Geometry: see drawing. Coordinates: mm, zero at the bounding-box minimum. A direction names the side the tool comes from. Coordinates: 2 decimals unless noted, no trailing zeros. Write each loop counter-clockwise with the first axis right and the second up, starting at its lowest first coordinate (ties: lowest second). Pieces come first, ordered by that corner, then holes. Notation, with made-up numbers: M 85.5,31.25 L 98.5,31.25 A17 cw 98.5,46.25 Z; hole C 89.25,33 d10. An arc over 180 degrees is marked long. Answer as CSV lines item,"result". Start each with the question number.
1. Section B-B on y = 70. Return the cut outline in (x, z), plus the area to 3 significant figures.
2. Contact query for flat-ended pins moving along their axis: pin 1 Ø2 at (x, z) = (172.5, 100) entering from +Y; pin 2 Ø10 at (x, z) = (100.5, 121.5) entering from +Y. Output: stop coordinate, or through.
3. Section D-D on z = 123.5. Return the cut outline in (x, y), plus the area to 3 significant figures.
4. Reachability of the marked faces 1 and 2 from +Z, -Z, +X, -X, +Y, -Y: full face, straight path, thin tool, end or side. Return the list, or none.
5. Mould query, pull axis Z, two halves, no side actions, for the marked faces 3, 4, 5 and 6. Classes: pulls with the +Z half, pulls with the -Z half, needs draft (parallel to the pull), parting line crosses it, or undercut.
6. Section C-C on z = 88.9. Return the cut outline in (x, y).
7. Line query: probe 1 along X at (y, z) = (24, 88); probe 2 along Z at (x, y) = (192, 61); probe 3 along Z at (x, y) = (215, 23). Output: solid intervals per line, ascending. Write a range as [from, to].
8. Section A-A on x = 88.9. Return the cut outline in (y, z), plus the area to 3 significant figures.
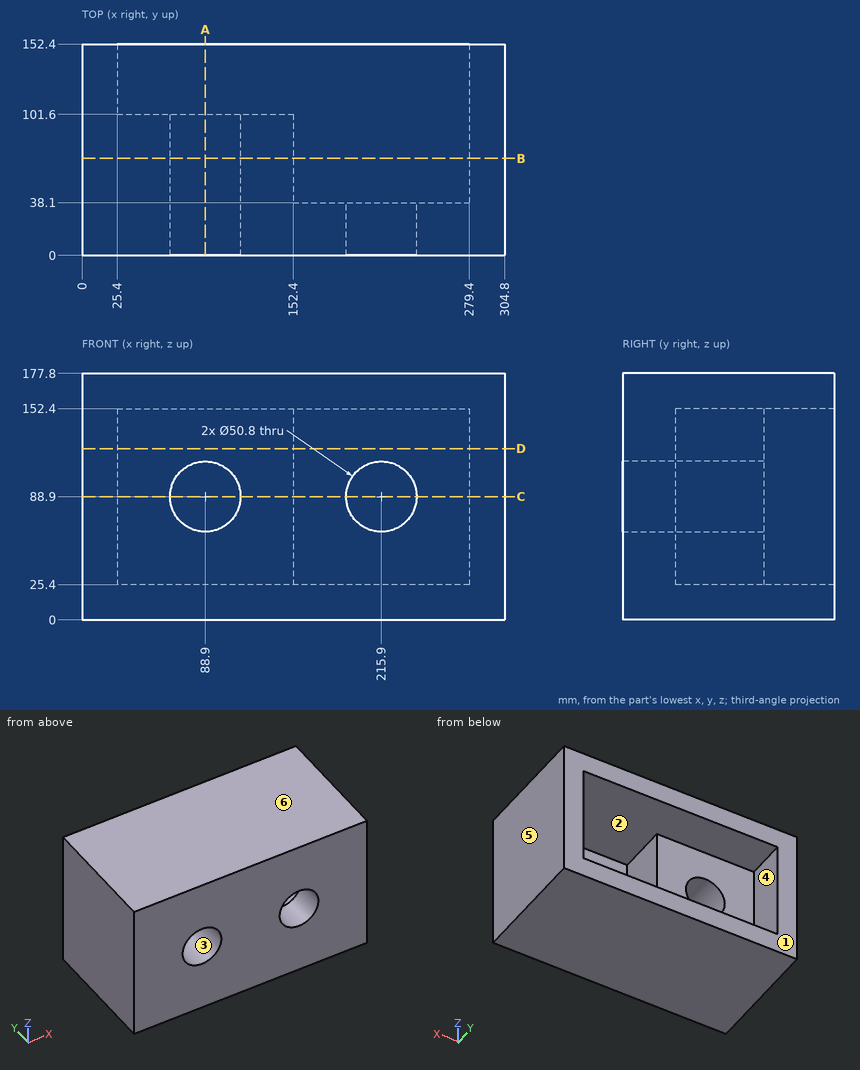
Values:
1,outline,"M 0,0 L 304.8,0 L 304.8,177.8 L 0,177.8 Z; hole C 88.9,88.9 d50.8; hole M 152.4,25.4 L 279.4,25.4 L 279.4,152.4 L 152.4,152.4 Z"
1,area,"36,000 mm²"
2,pin 1,"y = 38.1"
2,pin 2,"y = 101.6"
3,outline,"M 0,0 L 304.8,0 L 304.8,152.4 L 279.4,152.4 L 279.4,38.1 L 152.4,38.1 L 152.4,101.6 L 25.4,101.6 L 25.4,152.4 L 0,152.4 Z"
3,area,"25,500 mm²"
4,face 1,"+Z, -Z, +X, -X, +Y"
4,face 2,"+Y"
5,face 3,"undercut"
5,face 4,"undercut"
5,face 5,"needs draft"
5,face 6,"pulls with the +Z half"
6,outline,"M 0,0 L 63.5,0 L 63.5,101.6 L 25.4,101.6 L 25.4,152.4 L 0,152.4 Z; M 114.3,0 L 190.5,0 L 190.5,38.1 L 152.4,38.1 L 152.4,101.6 L 114.3,101.6 Z; M 241.3,0 L 304.8,0 L 304.8,152.4 L 279.4,152.4 L 279.4,38.1 L 241.3,38.1 Z"
7,probe 1,"[0, 63.52], [114.28, 190.52], [241.28, 304.8]"
7,probe 2,"[0, 25.4], [152.4, 177.8]"
7,probe 3,"[0, 63.52], [114.28, 177.8]"
8,outline,"M 0,0 L 152.4,0 L 152.4,25.4 L 101.6,25.4 L 101.6,63.5 L 0,63.5 Z; M 0,114.3 L 101.6,114.3 L 101.6,152.4 L 152.4,152.4 L 152.4,177.8 L 0,177.8 Z"
8,area,"15,500 mm²"
